Geometry: final body of the model. Coordinates: model frame, mm. A direction names the side the tool comes from. Give positions to 0.01 mm unless a question says otherwise; leave off trailing zeros. Order: outer loops, then holes, each group sorted by start corner. A loop starts at its lowest first (then second) coordinate and runs counter-clockwise, first axis right, second up. Notation, with made-up numbers: (37, -18.5) -> (95, -18.5) arc R14 ccw to (95, 8.5) -> close; hole circle Ø7 at (47.5, 0.25). An arc over 180 degrees is marked (long way). One line per question, with ' | ' between items. Start each with the question number.
(1) Mould query, pull axis Z, two halves, no side actions, for faces 1 (the face through (5, 10, 20)), 2 (the face through (6.591, 50.727, 18.358)), 3 (the face through (12, 70, 11)). Classes: +Z half, -Z half, draft (parallel to the pull), parting line (faces both ways), or undercut.
(2) Set-up query: faces 4 (the face through (15, 35, 0)), 5 (the face through (16.21, 56.897, 8.07)). Return all of +Z, -Z, +X, -X, +Y, -Y with unobstructed straight access to the full face (end or side cutting, diameter ignored); none if empty.
(3) Section B-B (y = 34). Return loops of the section in (x, z), then the cut area to 3 significant figures.
(4) Section D-D (x = 11). Return loops of the section in (y, z).
(5) First-contact query: pin 1 Ø12 at (y, z) = (42, 23) entering from +X; pin 2 Ø8 at (y, z) = (47, 22) entering from +X; pin 3 Ø3.5 at (x, y) = (18, 20) entering from -Z; pin 4 Ø8 at (x, z) = (22.5, 23.5) entering from -Y. Flat tips, straight axial feed; report the tip coordinate or a pass-through.
(6) Section A-A (z = 4). Return loops of the section in (x, y).
(7) Ray query, L1, parallel to Z at x = 8.25, y = 20; L2, parallel to Y at x = 16, z = 3.5. Return the intervals inside material, ascending.
(8) Section C-C (z = 24). Return loops of the section in (x, y), then the cut area to 3 significant figures.
```python
from build123d import *

# Parameters (mm, degrees)
SCHIZZO1_W                   = 30
SCHIZZO1_H                   = 40
ESTRUSIONE_ESTRUSIONE1_DEPTH = 30
SMUSSO1_SIZE                 = 20
ESTRUSIONE_ESTRUSIONE2_DEPTH = 30
FORO_PER_VITE_M5_1_D         = 5.5
FORO_PER_VITE_M5_1_DEPTH     = 13
FORO_PER_VITE_M5_1_TIP       = 1.652366702
FORO_PER_VITE_M5_2_D         = 5.5
FORO_PER_VITE_M5_2_DEPTH     = 13
FORO_PER_VITE_M5_2_TIP       = 1.652366702
SCHIZZO6_R                   = 7.5
TAGLIO_ESTRUSIONE1_DEPTH     = 3
FORO_PER_VITE_M4_1_D         = 4.5
FORO_PER_VITE_M4_1_DEPTH     = 10
FORO_PER_VITE_M4_1_TIP       = 1.351936393


with BuildPart() as part:
    # Schizzo1 → Estrusione-Estrusione1 (new body)
    with BuildSketch(Plane.XY):
        with Locations((15, 20)):
            Rectangle(SCHIZZO1_W, SCHIZZO1_H)
    extrude(amount=ESTRUSIONE_ESTRUSIONE1_DEPTH)

    # Smusso1
    smusso1_edges = [part.edges().sort_by_distance(p)[0] for p in [
        (30, 20, 30),
        (30, 0, 15),
        (15, 0, 30),
    ]]
    chamfer(smusso1_edges, length=SMUSSO1_SIZE)

    # Schizzo2 → Estrusione-Estrusione2 (add)
    with BuildSketch(Plane(origin=(0, 40, 0), x_dir=(1, 0, 0), z_dir=(0, 1, 0))):
        Polygon((0, 0), (30, 0), (30, -10), (10, -30), (0, -30), align=None)
    extrude(amount=ESTRUSIONE_ESTRUSIONE2_DEPTH)

    # Foro per Vite M5-1
    with Locations(Plane.ZY):
        with Locations((18, 20), (18, 48)):
            Hole(FORO_PER_VITE_M5_1_D / 2, depth=FORO_PER_VITE_M5_1_DEPTH)
            with Locations((0, 0, -(FORO_PER_VITE_M5_1_DEPTH + FORO_PER_VITE_M5_1_TIP / 2))):  # 118° drill point
                Cone(0, FORO_PER_VITE_M5_1_D / 2, FORO_PER_VITE_M5_1_TIP, mode=Mode.SUBTRACT)

    # Foro per Vite M5-2
    with Locations(Plane(origin=(18, 20, 0), x_dir=(-1, 0, 0), z_dir=(0, 0, -1))):
        with Locations((0, 0)):
            Hole(FORO_PER_VITE_M5_2_D / 2, depth=FORO_PER_VITE_M5_2_DEPTH)
            with Locations((0, 0, -(FORO_PER_VITE_M5_2_DEPTH + FORO_PER_VITE_M5_2_TIP / 2))):  # 118° drill point
                Cone(0, FORO_PER_VITE_M5_2_D / 2, FORO_PER_VITE_M5_2_TIP, mode=Mode.SUBTRACT)

    # Schizzo6 → Taglio-Estrusione1 (cut)
    with BuildSketch(Plane(origin=(0, 0, 0), x_dir=(-1, 0, 0), z_dir=(0, 0, -1))):
        with Locations((-15, 55)):
            Circle(SCHIZZO6_R)
    extrude(amount=-TAGLIO_ESTRUSIONE1_DEPTH, mode=Mode.SUBTRACT)

    # Foro per Vite M4-1
    with Locations(Plane(origin=(0, 0, 3), x_dir=(-1, 0, 0), z_dir=(0, 0, -1))):
        with Locations((-15, 55)):
            Hole(FORO_PER_VITE_M4_1_D / 2, depth=FORO_PER_VITE_M4_1_DEPTH)
            with Locations((0, 0, -(FORO_PER_VITE_M4_1_DEPTH + FORO_PER_VITE_M4_1_TIP / 2))):  # 118° drill point
                Cone(0, FORO_PER_VITE_M4_1_D / 2, FORO_PER_VITE_M4_1_TIP, mode=Mode.SUBTRACT)


solid = part.part
```
Response:
1) face 1: +Z half | face 2: undercut | face 3: draft
2) face 4: -Z, +X, -X, +Y, -Y | face 5: -Z
3) outline: (0, 0) -> (30, 0) -> (30, 10) -> (10, 30) -> (0, 30) -> close | area: 700 mm^2
4) outline: (1, 0) -> (48.66, 0) -> (48.66, 3) -> (61.34, 3) -> (61.34, 0) -> (70, 0) -> (70, 29) -> (20, 29) -> (1, 10) -> close; hole circle Ø5.5 at (20, 18); hole circle Ø5.5 at (48, 18)
5) pin 1: stops at x = 23 | pin 2: stops at x = 22 | pin 3: stops at z = 13.6 | pin 4: passes through
6) outline: (0, 0) -> (10, 0) -> (30, 20) -> (30, 70) -> (0, 70) -> close; hole circle Ø4.5 at (15, 55); hole circle Ø5.5 at (18, 20)
7) L1: z = 0 to 15.25, 20.75 to 30 | L2: y = 6 to 18.11, 21.89 to 52.98, 57.02 to 70
8) outline: (0, 14) -> (10, 14) -> (16, 20) -> (16, 70) -> (0, 70) -> close | area: 878 mm^2
